Answer from the drawing. Dimensions are ordinates in mm from the lowest x, y and z of the part. A direction names the side the tool comes from. Round coordinates to 2 decimals unless told otherwise and drop trailing zeros. Loops run counter-clockwise (first coordinate to the right, second up) from the corner with the lowest first, then second, coordinate; pieces in that order, holes last. Notation, with made-up numbers: (75.25, 22.5) - (105.25, 22.5) arc R28 cw to (105.25, 48.5) - close; hole circle Ø3 at (28.5, -2.5). An arc over 180 degrees is marked (long way). Write item = value, one per line. Start each with the question number.
1) A tool of negligible diameter and unlimited length cuts with its end or side. For the marked faces 1 and 2, from which of +Z, -Z, +X, -X, +Y, -Y can it reach the whole face along a straight path? Write none if from no direction.
2) Section B-B, the plane x = 13 is taken. Determine the outline of the cut face in (y, z).
3) Section C-C, the plane x = 8 is taken. Determine the outline of the cut face in (y, z).
4) Section A-A, the plane y = 20 is taken. Determine the outline of the cut face in (x, z).
5) Given pin 1 Ø2.5 at (y, z) = (30, 1.5) entering from -X; pin 2 Ø3 at (x, y) = (13, 47) entering from +Z, each flat-ended and moving along its own axis, determine where each tip first touches the part or whether it passes through.
6) Straight lines are drawn through the part: line 1 along Y through (x, z) = (5, 2); line 2 along X through (y, z) = (17.5, 2); line 3 along Y through (x, z) = (7.5, 2). For each, find the intervals that lie inside material, in ascending order.
7) Section D-D, the plane y = 47 is taken. Determine the outline of the cut face in (x, z).
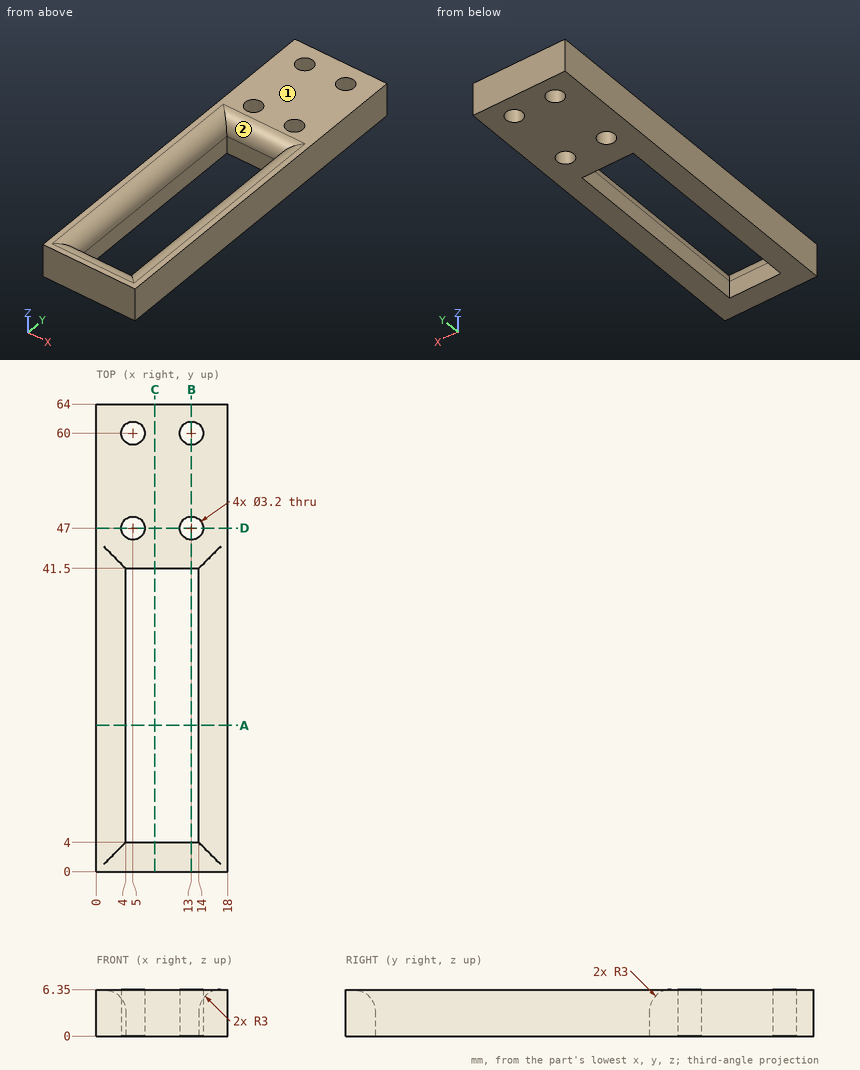
Geometry check:
q1.face_1 = +Z, +X, -X, +Y, -Y
q1.face_2 = +Z
q2.outline = (0, 0) - (4, 0) - (4, 3.35) arc R3 ccw to (1, 6.35) - (0, 6.35) - close; (41.5, 0) - (45.4, 0) - (45.4, 6.35) - (44.5, 6.35) arc R3 ccw to (41.5, 3.35) - close; (48.6, 0) - (58.4, 0) - (58.4, 6.35) - (48.6, 6.35) - close; (61.6, 0) - (64, 0) - (64, 6.35) - (61.6, 6.35) - close
q3.outline = (0, 0) - (4, 0) - (4, 3.35) arc R3 ccw to (1, 6.35) - (0, 6.35) - close; (41.5, 0) - (64, 0) - (64, 6.35) - (44.5, 6.35) arc R3 ccw to (41.5, 3.35) - close
q4.outline = (0, 0) - (4, 0) - (4, 3.35) arc R3 ccw to (1, 6.35) - (0, 6.35) - close; (14, 0) - (18, 0) - (18, 6.35) - (17, 6.35) arc R3 ccw to (14, 3.35) - close
q5.pin_1 = 0
q5.pin_2 = through
q6.line_1 = 0 to 4, 41.5 to 45.4, 48.6 to 58.4, 61.6 to 64
q6.line_2 = 0 to 4, 14 to 18
q6.line_3 = 0 to 4, 41.5 to 64
q7.outline = (0, 0) - (3.4, 0) - (3.4, 6.35) - (0, 6.35) - close; (6.6, 0) - (11.4, 0) - (11.4, 6.35) - (6.6, 6.35) - close; (14.6, 0) - (18, 0) - (18, 6.35) - (14.6, 6.35) - close
